```python
from build123d import *

# Parameters (mm, degrees)
EXTRUDE_1_DEPTH     = 199
CUT_EXTRUDE_1_DEPTH = 195
SKETCH_4_W          = 8
SKETCH_4_H          = 198
EXTRUDE_2_DEPTH     = 195
FILLET_1_R          = 2
CUT_EXTRUDE_2_REACH = 343.921
SKETCH_6_R          = 2
SKETCH_6_R_2        = 9
CUT_EXTRUDE_3_REACH = 297.87
SKETCH_7_R          = 9
FILLET_2_R          = 2
CUT_EXTRUDE_4_REACH = 442.798
SKETCH_9_R          = 9
CUT_EXTRUDE_5_REACH = 343.921
SKETCH_11_R         = 1.6
CUT_EXTRUDE_6_REACH = 343.921
SKETCH_12_R         = 1.6
CUT_EXTRUDE_7_REACH = 343.921
SKETCH_13_R         = 2.5


with BuildPart() as part:
    # 草图1 → 凸台-拉伸1 (new body)
    with BuildSketch(Plane(origin=(0, 0, 0), x_dir=(1, 0, 0), z_dir=(0, 1, 0))):
        with BuildLine():
            Line((-167, 101.5), (167, 101.5))
            ThreePointArc((167, 101.5), (183.263455967, 94.763455967), (190, 78.5))
            Line((190, 78.5), (190, -78.5))
            ThreePointArc((190, -78.5), (183.263455967, -94.763455967), (167, -101.5))
            Line((167, -101.5), (-167, -101.5))
            ThreePointArc((-167, -101.5), (-183.263455967, -94.763455967), (-190, -78.5))
            Line((-190, -78.5), (-190, 78.5))
            ThreePointArc((-190, 78.5), (-183.263455967, 94.763455967), (-167, 101.5))
        make_face()
    extrude(amount=EXTRUDE_1_DEPTH)

    # 草图3 → 切除-拉伸1 (cut)
    with BuildSketch(Plane(origin=(0, 199, 0), x_dir=(1, 0, 0), z_dir=(0, 1, 0))):
        with BuildLine():
            Line((-167, 99), (167, 99))
            ThreePointArc((167, 99), (181.495689014, 92.995689014), (187.5, 78.5))
            Line((187.5, 78.5), (187.5, -78.5))
            ThreePointArc((187.5, -78.5), (181.495689014, -92.995689014), (167, -99))
            Line((167, -99), (-167, -99))
            ThreePointArc((-167, -99), (-181.495689014, -92.995689014), (-187.5, -78.5))
            Line((-187.5, -78.5), (-187.5, 78.5))
            ThreePointArc((-187.5, 78.5), (-181.495689014, 92.995689014), (-167, 99))
        make_face()
    extrude(amount=-CUT_EXTRUDE_1_DEPTH, mode=Mode.SUBTRACT)

    # 草图4 → 凸台-拉伸2 (add)
    with BuildSketch(Plane(origin=(0, 4, 0), x_dir=(1, 0, 0), z_dir=(0, 1, 0))):
        Rectangle(SKETCH_4_W, SKETCH_4_H)
    extrude(amount=EXTRUDE_2_DEPTH)

    # 圆角1
    fillet_1_edges = [part.edges().sort_by_distance(p)[0] for p in [
        (-181.495689014, 4, 92.995689014),
        (-187.5, 4, 0),
        (-181.495689014, 4, -92.995689014),
        (85.5, 4, -99),
        (181.495689014, 4, -92.995689014),
        (187.5, 4, 0),
        (181.495689014, 4, 92.995689014),
        (-85.5, 4, 99),
        (85.5, 4, 99),
        (-85.5, 4, -99),
        (4, 101.5, -99),
        (-4, 4, 0),
        (-4, 101.5, -99),
        (-4, 101.5, 99),
        (4, 4, 0),
        (4, 101.5, 99),
    ]]
    fillet(fillet_1_edges, radius=FILLET_1_R)

    # 草图6 → 切除-拉伸2 (cut, up to next)
    with BuildSketch(Plane(origin=(0, 0, -101.5), x_dir=(-1, 0, 0), z_dir=(0, 0, -1)), mode=Mode.PRIVATE) as cut_extrude_2_sk1:
        with Locations((-155, 119)):
            Circle(SKETCH_6_R)
    cut_extrude_2_tool1 = extrude(cut_extrude_2_sk1.sketch, amount=-CUT_EXTRUDE_2_REACH, mode=Mode.PRIVATE) & part.part
    # 草图6 → 切除-拉伸2 (cut, up to next)
    with BuildSketch(Plane(origin=(0, 0, -101.5), x_dir=(-1, 0, 0), z_dir=(0, 0, -1)), mode=Mode.PRIVATE) as cut_extrude_2_sk2:
        with Locations((-155, 64)):
            Circle(SKETCH_6_R)
    cut_extrude_2_tool2 = extrude(cut_extrude_2_sk2.sketch, amount=-CUT_EXTRUDE_2_REACH, mode=Mode.PRIVATE) & part.part
    # 草图6 → 切除-拉伸2 (cut, up to next)
    with BuildSketch(Plane(origin=(0, 0, -101.5), x_dir=(-1, 0, 0), z_dir=(0, 0, -1)), mode=Mode.PRIVATE) as cut_extrude_2_sk3:
        with Locations((-78.5, 64)):
            Circle(SKETCH_6_R)
    cut_extrude_2_tool3 = extrude(cut_extrude_2_sk3.sketch, amount=-CUT_EXTRUDE_2_REACH, mode=Mode.PRIVATE) & part.part
    # 草图6 → 切除-拉伸2 (cut, up to next)
    with BuildSketch(Plane(origin=(0, 0, -101.5), x_dir=(-1, 0, 0), z_dir=(0, 0, -1)), mode=Mode.PRIVATE) as cut_extrude_2_sk4:
        with Locations((-78.5, 119)):
            Circle(SKETCH_6_R)
    cut_extrude_2_tool4 = extrude(cut_extrude_2_sk4.sketch, amount=-CUT_EXTRUDE_2_REACH, mode=Mode.PRIVATE) & part.part
    # 草图6 → 切除-拉伸2 (cut, up to next)
    with BuildSketch(Plane(origin=(0, 0, -101.5), x_dir=(-1, 0, 0), z_dir=(0, 0, -1)), mode=Mode.PRIVATE) as cut_extrude_2_sk5:
        with Locations((-31, 169)):
            Circle(SKETCH_6_R_2)
    cut_extrude_2_tool5 = extrude(cut_extrude_2_sk5.sketch, amount=-CUT_EXTRUDE_2_REACH, mode=Mode.PRIVATE) & part.part
    add(cut_extrude_2_tool1.solids().sort_by_distance((155, 119, -101.5))[0], mode=Mode.SUBTRACT)
    add(cut_extrude_2_tool2.solids().sort_by_distance((155, 64, -101.5))[0], mode=Mode.SUBTRACT)
    add(cut_extrude_2_tool3.solids().sort_by_distance((78.5, 64, -101.5))[0], mode=Mode.SUBTRACT)
    add(cut_extrude_2_tool4.solids().sort_by_distance((78.5, 119, -101.5))[0], mode=Mode.SUBTRACT)
    add(cut_extrude_2_tool5.solids().sort_by_distance((31, 169, -101.5))[0], mode=Mode.SUBTRACT)

    # 草图7 → 切除-拉伸3 (cut, up to next)
    with BuildSketch(Plane(origin=(4, 0, 0), x_dir=(0, 0, -1), z_dir=(1, 0, 0)), mode=Mode.PRIVATE) as cut_extrude_3_sk1:
        with Locations((64, 169)):
            Circle(SKETCH_7_R)
    cut_extrude_3_tool1 = extrude(cut_extrude_3_sk1.sketch, amount=-CUT_EXTRUDE_3_REACH, mode=Mode.PRIVATE) & part.part
    add(cut_extrude_3_tool1.solids().sort_by_distance((4, 169, -64))[0], mode=Mode.SUBTRACT)

    # 圆角2
    fillet_2_edges = [part.edges().sort_by_distance(p)[0] for p in [
        (-4, 169, -55),
        (4, 169, -55),
    ]]
    fillet(fillet_2_edges, radius=FILLET_2_R)

    # 草图9 → 切除-拉伸4 (cut, up to next)
    with BuildSketch(Plane(origin=(190, 0, 0), x_dir=(0, 0, -1), z_dir=(1, 0, 0)), mode=Mode.PRIVATE) as cut_extrude_4_sk1:
        with Locations((53.5, 169)):
            Circle(SKETCH_9_R)
    cut_extrude_4_tool1 = extrude(cut_extrude_4_sk1.sketch, amount=-CUT_EXTRUDE_4_REACH, mode=Mode.PRIVATE) & part.part
    add(cut_extrude_4_tool1.solids().sort_by_distance((190, 169, -53.5))[0], mode=Mode.SUBTRACT)

    # 草图11 → 切除-拉伸5 (cut, up to next)
    with BuildSketch(Plane.XY.offset(101.5), mode=Mode.PRIVATE) as cut_extrude_5_sk1:
        with Locations((77, 179)):
            Circle(SKETCH_11_R)
    cut_extrude_5_tool1 = extrude(cut_extrude_5_sk1.sketch, amount=-CUT_EXTRUDE_5_REACH, mode=Mode.PRIVATE) & part.part
    # 草图11 → 切除-拉伸5 (cut, up to next)
    with BuildSketch(Plane.XY.offset(101.5), mode=Mode.PRIVATE) as cut_extrude_5_sk2:
        with Locations((147, 179)):
            Circle(SKETCH_11_R)
    cut_extrude_5_tool2 = extrude(cut_extrude_5_sk2.sketch, amount=-CUT_EXTRUDE_5_REACH, mode=Mode.PRIVATE) & part.part
    # 草图11 → 切除-拉伸5 (cut, up to next)
    with BuildSketch(Plane.XY.offset(101.5), mode=Mode.PRIVATE) as cut_extrude_5_sk3:
        with Locations((77, 109)):
            Circle(SKETCH_11_R)
    cut_extrude_5_tool3 = extrude(cut_extrude_5_sk3.sketch, amount=-CUT_EXTRUDE_5_REACH, mode=Mode.PRIVATE) & part.part
    # 草图11 → 切除-拉伸5 (cut, up to next)
    with BuildSketch(Plane.XY.offset(101.5), mode=Mode.PRIVATE) as cut_extrude_5_sk4:
        with Locations((147, 109)):
            Circle(SKETCH_11_R)
    cut_extrude_5_tool4 = extrude(cut_extrude_5_sk4.sketch, amount=-CUT_EXTRUDE_5_REACH, mode=Mode.PRIVATE) & part.part
    add(cut_extrude_5_tool1.solids().sort_by_distance((77, 179, 101.5))[0], mode=Mode.SUBTRACT)
    add(cut_extrude_5_tool2.solids().sort_by_distance((147, 179, 101.5))[0], mode=Mode.SUBTRACT)
    add(cut_extrude_5_tool3.solids().sort_by_distance((77, 109, 101.5))[0], mode=Mode.SUBTRACT)
    add(cut_extrude_5_tool4.solids().sort_by_distance((147, 109, 101.5))[0], mode=Mode.SUBTRACT)

    # 草图12 → 切除-拉伸6 (cut, up to next)
    with BuildSketch(Plane.XY.offset(101.5), mode=Mode.PRIVATE) as cut_extrude_6_sk1:
        with Locations((77, 144)):
            Circle(SKETCH_12_R)
    cut_extrude_6_tool1 = extrude(cut_extrude_6_sk1.sketch, amount=-CUT_EXTRUDE_6_REACH, mode=Mode.PRIVATE) & part.part
    # 草图12 → 切除-拉伸6 (cut, up to next)
    with BuildSketch(Plane.XY.offset(101.5), mode=Mode.PRIVATE) as cut_extrude_6_sk2:
        with Locations((112, 179)):
            Circle(SKETCH_12_R)
    cut_extrude_6_tool2 = extrude(cut_extrude_6_sk2.sketch, amount=-CUT_EXTRUDE_6_REACH, mode=Mode.PRIVATE) & part.part
    # 草图12 → 切除-拉伸6 (cut, up to next)
    with BuildSketch(Plane.XY.offset(101.5), mode=Mode.PRIVATE) as cut_extrude_6_sk3:
        with Locations((147, 144)):
            Circle(SKETCH_12_R)
    cut_extrude_6_tool3 = extrude(cut_extrude_6_sk3.sketch, amount=-CUT_EXTRUDE_6_REACH, mode=Mode.PRIVATE) & part.part
    # 草图12 → 切除-拉伸6 (cut, up to next)
    with BuildSketch(Plane.XY.offset(101.5), mode=Mode.PRIVATE) as cut_extrude_6_sk4:
        with Locations((112, 109)):
            Circle(SKETCH_12_R)
    cut_extrude_6_tool4 = extrude(cut_extrude_6_sk4.sketch, amount=-CUT_EXTRUDE_6_REACH, mode=Mode.PRIVATE) & part.part
    add(cut_extrude_6_tool1.solids().sort_by_distance((77, 144, 101.5))[0], mode=Mode.SUBTRACT)
    add(cut_extrude_6_tool2.solids().sort_by_distance((112, 179, 101.5))[0], mode=Mode.SUBTRACT)
    add(cut_extrude_6_tool3.solids().sort_by_distance((147, 144, 101.5))[0], mode=Mode.SUBTRACT)
    add(cut_extrude_6_tool4.solids().sort_by_distance((112, 109, 101.5))[0], mode=Mode.SUBTRACT)

    # 草图13 → 切除-拉伸7 (cut, up to next)
    with BuildSketch(Plane.XY.offset(101.5), mode=Mode.PRIVATE) as cut_extrude_7_sk1:
        with Locations((99, 42.5)):
            Circle(SKETCH_13_R)
    cut_extrude_7_tool1 = extrude(cut_extrude_7_sk1.sketch, amount=-CUT_EXTRUDE_7_REACH, mode=Mode.PRIVATE) & part.part
    # 草图13 → 切除-拉伸7 (cut, up to next)
    with BuildSketch(Plane.XY.offset(101.5), mode=Mode.PRIVATE) as cut_extrude_7_sk2:
        with Locations((151, 42.5)):
            Circle(SKETCH_13_R)
    cut_extrude_7_tool2 = extrude(cut_extrude_7_sk2.sketch, amount=-CUT_EXTRUDE_7_REACH, mode=Mode.PRIVATE) & part.part
    add(cut_extrude_7_tool1.solids().sort_by_distance((99, 42.5, 101.5))[0], mode=Mode.SUBTRACT)
    add(cut_extrude_7_tool2.solids().sort_by_distance((151, 42.5, 101.5))[0], mode=Mode.SUBTRACT)


solid = part.part
```
Could you check a few things on this model? Use its own coordinates, in mm. A direction names the side the tool comes from. Coordinates: 2 decimals unless noted, no trailing zeros. Write each loop counter-clockwise with the first axis right and the second up, starting at its lowest first coordinate (ties: lowest second). Pieces come first, ordered by that corner, then holes. Notation, with made-up numbers: (-30, 82.5) - (28, 82.5) arc R15 ccw to (28, 110.5) - close; hole circle Ø5 at (35.5, 69.5). An arc over 180 degrees is marked (long way). Use a Markdown table: item, result.
Q1. Imagine slicing it at D-D (x = 137). List the corners of the cut face in (y, z) for me, and give its area (3 significant figures).
Geometry check:
| item | result |
|---|---|
| outline | (0, -101.5) - (199, -101.5) - (199, -99) - (6, -99) arc R2 cw to (4, -97) - (4, 97) arc R2 cw to (6, 99) - (199, 99) - (199, 101.5) - (0, 101.5) - close |
| area | 1,790 mm2 |
Q2. Please list where these lines run through material, in increasing order: L1, parallel to X at y = 190.5, z = 26.5; L2, parallel to Y at x = 77, z = 100; L3, parallel to Z at x = -119, y = 188.
Geometry check:
| item | result |
|---|---|
| L1 | x = -190 to -187.5, -4 to 4, 187.5 to 190 |
| L2 | y = 0 to 107.4, 110.6 to 142.4, 145.6 to 177.4, 180.6 to 199 |
| L3 | z = -101.5 to -99, 99 to 101.5 |
Q3. Which directions (+Z, -Z, +X, -X, +Y, -Y) give clear straight access to the entire face, cutting with the end or side of a thin tool? Please do faces 1 (the cylindrical face through (0.03, 176.59, -68.84)), 2 (the flat face through (-187.5, 104, 1)), 3 (the cylindrical face through (188.768, 177.923, -52.328)).
Geometry check:
| item | result |
|---|---|
| face 1 | none |
| face 2 | +Y |
| face 3 | +X |
Q4. Imagine slicing it at C-C (z = 52.5). List the corners of the cut face in (x, y) for me.
Geometry check:
| item | result |
|---|---|
| outline | (-190, 0) - (190, 0) - (190, 199) - (187.5, 199) - (187.5, 6) arc R2 cw to (185.5, 4) - (6, 4) arc R2 cw to (4, 6) - (4, 199) - (-4, 199) - (-4, 6) arc R2 cw to (-6, 4) - (-185.5, 4) arc R2 cw to (-187.5, 6) - (-187.5, 199) - (-190, 199) - close |
Q5. I'm going to push flat-ended pins straight in: pin 1 Ø3 at (x, z) = (51.5, 19.5) entering from +Y; pin 2 Ø2.5 at (x, y) = (155, 64) entering from -Z; pin 3 Ø1.9 at (x, y) = (147, 179) entering from +Z. Where does each tip first touch, or does it pass through?
Geometry check:
| item | result |
|---|---|
| pin 1 | stops at y = 4 |
| pin 2 | stops at z = 99 |
| pin 3 | stops at z = -99 |
Q6. Imagine slicing it at B-B (x = 31). List the corners of the cut face in (y, z) for me.
Geometry check:
| item | result |
|---|---|
| outline | (0, -101.5) - (160, -101.5) - (160, -99) - (6, -99) arc R2 cw to (4, -97) - (4, 97) arc R2 cw to (6, 99) - (199, 99) - (199, 101.5) - (0, 101.5) - close; (178, -101.5) - (199, -101.5) - (199, -99) - (178, -99) - close |
Q7. Imagine slicing it at A-A (y = 51.5). List the corners of the cut face in (x, z) for me, and give its area (3 significant figures).
Geometry check:
| item | result |
|---|---|
| outline | (-190, -78.5) arc R23 ccw to (-167, -101.5) - (167, -101.5) arc R23 ccw to (190, -78.5) - (190, 78.5) arc R23 ccw to (167, 101.5) - (-167, 101.5) arc R23 ccw to (-190, 78.5) - close; hole (-187.5, -78.5) arc R20.5 ccw to (-167, -99) - (-6, -99) arc R2 ccw to (-4, -97) - (-4, 97) arc R2 ccw to (-6, 99) - (-167, 99) arc R20.5 ccw to (-187.5, 78.5) - close; hole (4, -97) arc R2 ccw to (6, -99) - (167, -99) arc R20.5 ccw to (187.5, -78.5) - (187.5, 78.5) arc R20.5 ccw to (167, 99) - (6, 99) arc R2 ccw to (4, 97) - close |
| area | 4,380 mm2 |
Q8. Thinking about a two-plate mould opening in Z: for faces 4 (the cylindrical face through (183.084, 98.107, -94.941)), 5 (the cylindrical face through (-183.084, 98.107, 94.941)), 6 (the flat face through (-88, 104, -99)), which applies, +Z half, -Z half, draft (parallel to the pull), parting line (faces both ways), or undercut?
Geometry check:
| item | result |
|---|---|
| face 4 | -Z half |
| face 5 | +Z half |
| face 6 | undercut |
